For this review, take the finished solid that the model builds, in its own axes (mm). A direction names the side the tool comes from. Coordinates: 2 decimals unless noted, no trailing zeros. Order: outer loops, then holes, each group sorted by start corner. A loop starts at its lowest first (then second) coordinate and runs counter-clockwise, first axis right, second up. Notation, with made-up numbers: M -8.75,79 L 36.25,79 A28 cw 36.25,98 Z; hole C -38,83.25 d11. An arc over 180 degrees is marked long. Use CSV: the item, a comma, the result in double quotes.
```python
from build123d import *

# Parameters (mm, degrees)
SKETCH_1_W                       = 35
SKETCH_1_H                       = 50
EXTRUDE_1_DEPTH                  = 2.5
SKETCH_2_R                       = 1.65
CUT_EXTRUDE_1_DEPTH              = 10
SM_EDGE_FLANGE_2_STRIP_W         = 14
SM_EDGE_FLANGE_2_STRIP_H         = 2.5
SM_EDGE_FLANGE_2_STRIP_CUT_DEPTH = 35
SM_EDGE_FLANGE_2_DEPTH           = 35
SKETCH_19_R                      = 3.5
EXTRUDE_2_DEPTH                  = 3
SKETCH_20_R                      = 1.65
CUT_EXTRUDE_2_DEPTH              = 10


# Sheet-metal steps are written as plain solids
with BuildPart() as part:
    # 草图1 → 凸台-拉伸1 (new body)
    with BuildSketch(Plane.XY):
        with Locations((17.5, 25)):
            Rectangle(SKETCH_1_W, SKETCH_1_H)
    extrude(amount=EXTRUDE_1_DEPTH)

    # 草图2 → 切除-拉伸1 (cut)
    with BuildSketch(Plane.XY.offset(2.5)):
        with Locations((7, 40.5)):
            Circle(SKETCH_2_R)
        with Locations((7, 10)):
            Circle(SKETCH_2_R)
    extrude(amount=-CUT_EXTRUDE_1_DEPTH, mode=Mode.SUBTRACT)

    # 边线-法兰2 strip (across the edge) → 边线-法兰2 strip cut (cut)
    with BuildSketch(Plane(origin=(0, 0, 2.5), x_dir=(0, 1, 0), z_dir=(1, 0, 0))):
        with Locations((-2.5, -1.25)):
            Rectangle(SM_EDGE_FLANGE_2_STRIP_W, SM_EDGE_FLANGE_2_STRIP_H)
    extrude(amount=SM_EDGE_FLANGE_2_STRIP_CUT_DEPTH, mode=Mode.SUBTRACT)

    # 边线-法兰2 section (across the edge) → 边线-法兰2 (add)
    with BuildSketch(Plane(origin=(0, 0, 2.5), x_dir=(0, 1, 0), z_dir=(1, 0, 0))):
        with BuildLine():
            Line((0, 2), (0, 12.5))
            Line((0, 12.5), (2.5, 12.5))
            Line((2.5, 12.5), (2.5, 2))
            ThreePointArc((2.5, 2), (3.085786438, 0.585786438), (4.5, 0))
            Line((4.5, 0), (4.5, -2.5))
            ThreePointArc((4.5, -2.5), (1.318019485, -1.181980515), (0, 2))
        make_face()
    extrude(amount=SM_EDGE_FLANGE_2_DEPTH)

    # 草图19 → 凸台-拉伸2 (add)
    with BuildSketch(Plane(origin=(0, 2.5, 0), x_dir=(1, 0, 0), z_dir=(0, 1, 0))):
        with Locations(Location((25, -10, 0), (0, 0, 270))):
            Circle(SKETCH_19_R)
    extrude(amount=EXTRUDE_2_DEPTH)

    # 草图20 → 切除-拉伸2 (cut)
    with BuildSketch(Plane(origin=(0, 5.5, 0), x_dir=(1, 0, 0), z_dir=(0, 1, 0))):
        with Locations(Location((25, -10, 0), (0, 0, 270))):
            Circle(SKETCH_20_R)
    extrude(amount=-CUT_EXTRUDE_2_DEPTH, mode=Mode.SUBTRACT)


solid = part.part
```
Item 1: Add section A-A on x = 7. State the section outline as (y, z) points, and give its area (3 significant figures).
Solutions:
outline,"M 0,4.5 A4.5 ccw 4.5,0 L 8.35,0 L 8.35,2.5 L 4.5,2.5 A2 cw 2.5,4.5 L 2.5,15 L 0,15 Z; M 11.65,0 L 38.85,0 L 38.85,2.5 L 11.65,2.5 Z; M 42.15,0 L 50,0 L 50,2.5 L 42.15,2.5 Z"
area,"136 mm^2"
Item 2: Draft analysis for pull direction Z (two halves, no side actions). For faces 1 (the face through (27.365, 3.979, 7.42)), 2 (the face through (17, 1, 15)), 3 (the face through (26.636, 2.788, 9.785)), 4 (the face through (17, 50, 1)), state which applies: released by +Z, released by -Z, zero draft, split by the parting line, or undercut.
Solutions:
face 1,"undercut"
face 2,"released by +Z"
face 3,"undercut"
face 4,"zero draft"
Item 3: Add section C-C on y = 10. State the section outline as (x, z) points, and give its area (4 significant figures).
Solutions:
outline,"M 0,0 L 5.35,0 L 5.35,2.5 L 0,2.5 Z; M 8.65,0 L 35,0 L 35,2.5 L 8.65,2.5 Z"
area,"79.25 mm^2"
Item 4: Add section D-D on x = 3.5. State the section outline as (y, z) points.
Solutions:
outline,"M 0,4.5 A4.5 ccw 4.5,0 L 50,0 L 50,2.5 L 4.5,2.5 A2 cw 2.5,4.5 L 2.5,15 L 0,15 Z"
Item 5: To check wall thickness, follow line 1 along X through (y, z) = (3.75, 10); line 2 along X through (y, z) = (2.45, 10); line 3 along Y through (x, z) = (7, 1.75). State the ranges of each line that lie inside material, in increasing order. Write a range as [from, to].
Solutions:
line 1,"[21.5, 23.35], [26.65, 28.5]"
line 2,"[0, 23.35], [26.65, 35]"
line 3,"[0.94, 8.35], [11.65, 38.85], [42.15, 50]"
Item 6: Clearance check with flat-ended pins moving along their axes: pin 1 Ø5 at (x, z) = (24.5, 11) entering from +Y; pin 2 Ø5 at (x, y) = (18, 36.5) entering from +Z. State where each tip first meets the part, or that it passes through.
Solutions:
pin 1,"y = 5.5"
pin 2,"z = 2.5"
Item 7: For faces 5 (the face through (24, 5.5, 12)), 6 (the face through (17.255, 1.353, 1.283)), list the 3-axis set-ups (+Z, -Z, +X, -X, +Y, -Y) from which the entire face can be reached by the end or side of a thin tool; tool diameter is ignored.
Solutions:
face 5,"+Z, +X, -X, +Y"
face 6,"-Z, +X, -X, -Y"
Item 8: Add section B-B on z = 10. State the section outline as (x, y) points, and give its area (4 significant figures).
Solutions:
outline,"M 0,0 L 23.35,0 L 23.35,5.5 L 21.5,5.5 L 21.5,2.5 L 0,2.5 Z; M 26.65,0 L 35,0 L 35,2.5 L 28.5,2.5 L 28.5,5.5 L 26.65,5.5 Z"
area,"90.35 mm^2"
